Input: part model. Units: mm. Frame: model coordinates. Coordinates: 2 decimals unless noted, no trailing zeros. Order: outer loops, then holes, each group sorted by start corner. A loop starts at its lowest first (then second) coordinate and runs counter-clockwise, first axis right, second up.
from build123d import *

# Parameters (mm, degrees)
SKIZZE2_W  = 19
SKIZZE2_H  = 2.5
FASE1_SIZE = 0.2


with BuildPart() as part:
    # Skizze2 → Rotation1 (revolve)
    with BuildSketch(Plane(origin=(0, 0, 0), x_dir=(1, 0, 0), z_dir=(0, 1, 0)), mode=Mode.PRIVATE) as rotation1_sk:
        with Locations((9.5, 6.25)):
            Rectangle(SKIZZE2_W, SKIZZE2_H)
        with Locations((9.5, -6.25)):
            Rectangle(SKIZZE2_W, SKIZZE2_H)
    revolve(rotation1_sk.sketch.rotate(Axis((0, 0, 0), (1, 0, 0)), 180), axis=Axis((0, 0, 0), (1, 0, 0)))

    # Fase1
    fase1_edges = [part.edges().sort_by_distance(p)[0] for p in [
        (0, 0, -5),
        (19, 0, -5),
        (19, 0, -7.5),
        (0, 0, -7.5),
    ]]
    chamfer(fase1_edges, length=FASE1_SIZE)


solid = part.part
Item 1: Pin query (flat end, axial travel): pin 1 Ø6 at (x, z) = (11.5, 5.5) entering from -Y; pin 2 Ø1 at (x, y) = (2, 3) entering from +Z; pin 3 Ø3 at (x, z) = (14.5, -2) entering from +Y. Return the tip coordinate at first contact, or that it passes through.
Response values:
pin 1: stops at y = -7.07
pin 2: stops at z = 7.07
pin 3: stops at y = 7.48
Item 2: Cut plane A-A on y = 0. Return loops of the section in (x, z).
Response values:
outline: (0, -7.3) - (0.2, -7.5) - (18.8, -7.5) - (19, -7.3) - (19, -5.2) - (18.8, -5) - (0.2, -5) - (0, -5.2) - close; (0, 5.2) - (0.2, 5) - (18.8, 5) - (19, 5.2) - (19, 7.3) - (18.8, 7.5) - (0.2, 7.5) - (0, 7.3) - close
Item 3: Cut plane C-C on x = 10.75. Return loops of the section in (y, z).
Response values:
outline: circle Ø15 at (0, 0); hole circle Ø10 at (0, 0)
Item 4: Ray query, probe 1 along Y at (x, z) = (5, 0); probe 2 along Z at (x, y) = (4.75, -3). Return the intervals inside material, ascending.
Response values:
probe 1: y = -7.5 to -5, 5 to 7.5
probe 2: z = -6.87 to -4, 4 to 6.87
Item 5: Draft query along Y for faces 1 (the face through (9.63, 6.324, -4.032)), 2 (the face through (10, 0, 5)), 3 (the face through (0, 2, 5)). Return one class per face: pulls with the +Y half, pulls with the -Y half, needs draft (parallel to the pull), parting line crosses it, or undercut.
Response values:
face 1: parting line crosses it
face 2: undercut
face 3: needs draft
